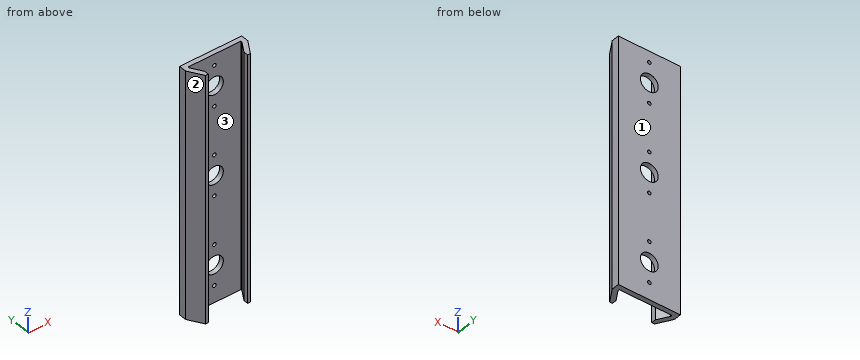
from build123d import *

# Parameters (mm, degrees)
BOSS_EXTRUDE1_DEPTH        = 213
SKETCH2_R                  = 7.5
CUT_EXTRUDE1_DEPTH         = 213
SKETCH7_R                  = 1.5
CUT_EXTRUDE2_DEPTH         = 10
LPATTERN1_COUNT            = 3
LPATTERN1_PITCH            = 75
SZKIC1_W                   = 52.4
SZKIC1_H                   = 5
WYTNIJ_WYCI_GNI_CIE1_DEPTH = 30.5


with BuildPart() as part:
    # Sketch1 → Boss-Extrude1 (new body)
    with BuildSketch(Plane.XY):
        Polygon((0, -13.289354466), (-22.2, -13.289354466), (-22.2, -14.545627613), (-16.612166923, -23.689354466), (-16.612166923, -27.689354466), (-18.855505392, -27.689354466), (-26.2, -15.671090562), (-26.2, -9.289354466), (26.2, -9.289354466), (26.2, -15.671090562), (18.855505392, -27.689354466), (16.612166923, -27.689354466), (16.612166923, -23.689354466), (22.2, -14.545627613), (22.2, -13.289354466), align=None)
    extrude(amount=BOSS_EXTRUDE1_DEPTH)

    # Sketch2 → Cut-Extrude1 (cut)
    with BuildSketch(Plane(origin=(0, -9.289354466, 0), x_dir=(1, 0, 0), z_dir=(0, 1, 0))):
        with Locations(Location((0, -31.5, 0), (0, 0, 180))):
            Circle(SKETCH2_R)
        with Locations(Location((0, -106.5, 0), (0, 0, 180))):
            Circle(SKETCH2_R)
        with Locations(Location((0, -181.5, 0), (0, 0, 180))):
            Circle(SKETCH2_R)
    extrude(amount=-CUT_EXTRUDE1_DEPTH, mode=Mode.SUBTRACT)

    # Sketch7 → Cut-Extrude2 (cut)
    with BuildSketch(Plane(origin=(0, -9.289354466, 0), x_dir=(1, 0, 0), z_dir=(0, 1, 0))):
        with Locations(Location((0, -198.624297731, 0), (0, 0, 180))):
            Circle(SKETCH7_R)
        with Locations(Location((0, -164.375702269, 0), (0, 0, 180))):
            Circle(SKETCH7_R)
    cut_extrude2 = extrude(amount=-CUT_EXTRUDE2_DEPTH, mode=Mode.SUBTRACT)

    # LPattern1: Cut-Extrude2 ×3
    with Locations(*[(0, 0, -i * LPATTERN1_PITCH) for i in range(1, LPATTERN1_COUNT)]):
        add(cut_extrude2, mode=Mode.SUBTRACT)

    # Szkic1 → Wytnij-wyciągnięcie1 (cut)
    with BuildSketch(Plane(origin=(0, -9.289354466, 0), x_dir=(1, 0, 0), z_dir=(0, 1, 0))):
        with Locations((0, -210.5)):
            Rectangle(SZKIC1_W, SZKIC1_H)
    extrude(amount=-WYTNIJ_WYCI_GNI_CIE1_DEPTH, mode=Mode.SUBTRACT)


solid = part.part
CAD build for the part. Positions are in the model's coordinates, mm. Face numbers are marked on the shaded views. Give positions to 0.01 mm unless a question says otherwise; leave off trailing zeros. Loops run counter-clockwise (first coordinate to the right, second up) from the corner with the lowest first, then second, coordinate; pieces in that order, holes last. Notation, with made-up numbers: M 80,-24 L 98,-24 A20 cw 98,14 Z; hole C -35.5,37 d7. An arc over 180 degrees is marked long. One line per question, with ' | ' between items. Start each with the question number.
1. Saw through at B-B on z = 31.5. Give the cut face in (x, y).
2. Saw through at C-C on z = 127.5. Give the cut face in (x, y), plus the area to 3 significant figures.
3. Saw through at A-A on x = -4.5. Give the cut face in (y, z), plus the area to 3 significant figures.
4. Saw through at D-D on y = -20.5. Give the cut face in (x, z).
5. Flat gauge pins, fed straight in: pin 1 (2 mm diameter, centred on y = -25.5, z = 119.5, fed in from -X); pin 2 (9 mm diameter, centred on x = 0, z = 31.5, fed in from +Y); pin 3 (3.5 mm diameter, centred on x = 0, z = 164.38, fed in from -Y); pin 4 (2 mm diameter, centred on y = -18, z = 91.5, fed in from -X). Where does each tip first touch, or does it go through?
6. Probe L1, parallel to X at y = -21.75, z = 145.5; L2, parallel to Z at x = 3.5, y = -12.75; L3, parallel to Y at x = 21, z = 110. List the from-to ranges inside material, lowest first. Write a range as from..to.
7. Two-plate mould, pull along X, no slides. Class the marked faces 1, 2 and 3: pulls with the +X half, pulls with the -X half, needs draft (parallel to the pull), parting line crosses it, or undercut.
Result sheet:
1) outline: M -26.2,-15.67 L -18.86,-27.69 L -16.61,-27.69 L -16.61,-23.69 L -22.2,-14.55 L -22.2,-13.29 L -7.5,-13.29 L -7.5,-9.29 L -26.2,-9.29 Z; M 7.5,-13.29 L 22.2,-13.29 L 22.2,-14.55 L 16.61,-23.69 L 16.61,-27.69 L 18.86,-27.69 L 26.2,-15.67 L 26.2,-9.29 L 7.5,-9.29 Z
2) outline: M -26.2,-15.67 L -18.86,-27.69 L -16.61,-27.69 L -16.61,-23.69 L -22.2,-14.55 L -22.2,-13.29 L 22.2,-13.29 L 22.2,-14.55 L 16.61,-23.69 L 16.61,-27.69 L 18.86,-27.69 L 26.2,-15.67 L 26.2,-9.29 L -26.2,-9.29 Z | area: 332 mm^2
3) outline: M -13.29,0 L -9.29,0 L -9.29,25.5 L -13.29,25.5 Z; M -13.29,37.5 L -9.29,37.5 L -9.29,100.5 L -13.29,100.5 Z; M -13.29,112.5 L -9.29,112.5 L -9.29,175.5 L -13.29,175.5 Z; M -13.29,187.5 L -9.29,187.5 L -9.29,208 L -13.29,208 Z | area: 688 mm^2
4) outline: M -23.25,0 L -18.56,0 L -18.56,208 L -23.25,208 Z; M 18.56,0 L 23.25,0 L 23.25,208 L 18.56,208 Z
5) pin 1: stops at x = -20.8 | pin 2: passes through | pin 3: stops at y = -13.29 | pin 4: stops at x = -25.39
6) L1: x = -22.49..-17.8, 17.8..22.49 | L2: z = 0..24.87, 38.13..99.87, 113.13..174.87, 188.13..208 | L3: y = -24.18..-16.51, -13.29..-9.29
7) face 1: needs draft | face 2: pulls with the -X half | face 3: undercut
